from build123d import *

# Parameters (mm, degrees)
SKETCH1_W                       = 110
SKETCH1_H                       = 42
BOSS_EXTRUDE1_DEPTH             = 10
CBORE_FOR_M3_SBHCS1_D           = 3.4
CBORE_FOR_M3_SBHCS1_CBORE_D     = 8
CBORE_FOR_M3_SBHCS1_CBORE_DEPTH = 5
CUT_EXTRUDE1_DEPTH              = 10
FILLET2_R                       = 5
SKETCH6_W                       = 110
SKETCH6_H                       = 18
BOSS_EXTRUDE2_DEPTH             = 40
BOSS_EXTRUDE3_DEPTH             = 5
BOSS_EXTRUDE4_DEPTH             = 5
SKETCH10_W                      = 35
SKETCH10_H                      = 13
CUT_EXTRUDE2_DEPTH              = 15
FILLET3_R                       = 5


with BuildPart() as part:
    # Sketch1 → Boss-Extrude1 (new body)
    with BuildSketch(Plane(origin=(0, 0, 0), x_dir=(1, 0, 0), z_dir=(0, 1, 0))):
        Rectangle(SKETCH1_W, SKETCH1_H)
    extrude(amount=BOSS_EXTRUDE1_DEPTH)

    # CBORE for M3 SBHCS1 (through all)
    with Locations(Plane(origin=(0, 10, 0), x_dir=(1, 0, 0), z_dir=(0, 1, 0))):
        with Locations((-45, 8), (-32, 3), (32, 3), (45, 8)):
            CounterBoreHole(CBORE_FOR_M3_SBHCS1_D / 2, CBORE_FOR_M3_SBHCS1_CBORE_D / 2, CBORE_FOR_M3_SBHCS1_CBORE_DEPTH)

    # Sketch4 → Cut-Extrude1 (cut)
    with BuildSketch(Plane(origin=(0, 10, 0), x_dir=(1, 0, 0), z_dir=(0, 1, 0))):
        with BuildLine():
            Line((24, -21), (24, 6))
            ThreePointArc((24, 6), (22.535533906, 9.535533906), (19, 11))
            Line((19, 11), (-6, 11))
            ThreePointArc((-6, 11), (-9.535533906, 9.535533906), (-11, 6))
            Line((-11, 6), (-11, -21))
            Line((-11, -21), (24, -21))
        make_face()
    extrude(amount=-CUT_EXTRUDE1_DEPTH, mode=Mode.SUBTRACT)

    # Fillet2
    fillet2_edges = [part.edges().sort_by_distance(p)[0] for p in [
        (-11, 5, 21),
        (24, 5, 21),
    ]]
    fillet(fillet2_edges, radius=FILLET2_R)

    # Sketch6 → Boss-Extrude2 (add)
    with BuildSketch(Plane(origin=(0, 10, 0), x_dir=(1, 0, 0), z_dir=(0, 1, 0))):
        with Locations((0, -12)):
            Rectangle(SKETCH6_W, SKETCH6_H)
    extrude(amount=BOSS_EXTRUDE2_DEPTH)

    # Sketch8 → Boss-Extrude3 (add)
    with BuildSketch(Plane.ZY.offset(55)):
        Polygon((-21, 10), (3, 10), (3, 50), align=None)
    extrude(amount=-BOSS_EXTRUDE3_DEPTH)

    # Sketch9 → Boss-Extrude4 (add)
    with BuildSketch(Plane(origin=(55, 0, 0), x_dir=(0, 0, -1), z_dir=(1, 0, 0))):
        Polygon((-3, 10), (21, 10), (-3, 50), align=None)
    extrude(amount=-BOSS_EXTRUDE4_DEPTH)

    # Sketch10 → Cut-Extrude2 (cut)
    with BuildSketch(Plane.XZ.offset(-10)):
        with Locations((6.5, 9.5)):
            Rectangle(SKETCH10_W, SKETCH10_H)
    extrude(amount=-CUT_EXTRUDE2_DEPTH, mode=Mode.SUBTRACT)

    # Fillet3
    fillet3_edges = [part.edges().sort_by_distance(p)[0] for p in [
        (24, 17.5, 3),
        (6.5, 25, 3),
        (-11, 17.5, 3),
    ]]
    fillet(fillet3_edges, radius=FILLET3_R)


solid = part.part
Here's how the part is built. I have some questions about the finished solid (model axes, mm). A direction names the side the tool comes from. Coordinates: 2 decimals unless noted, no trailing zeros. Order: outer loops, then holes, each group sorted by start corner. A loop starts at its lowest first (then second) coordinate and runs counter-clockwise, first axis right, second up. Notation, with made-up numbers: M 47.5,17 L 66.5,17 A12 ccw 66.5,27 Z; hole C 23.25,86.25 d11. An arc over 180 degrees is marked long. Answer as CSV lines item,"result". Start each with the question number.
1. I want a section at B-B, the plane x = -32. Write out the boundary of the cut face in (y, z).
2. On a 3-axis mill with a long thin cutter (end or side, diameter ignored), from which of +Z, -Z, +X, -X, +Y, -Y can I reach the whole of each face in a straight line? I mean faces 4 (the flat face through (7, 5, -11)), 5 (the flat face through (-11, 7, 7)), 6 (the flat face through (6, 17, 16)), 7 (the flat face through (34, 5, -3)). Say none if no direction works.
3. I want a section at D-D, the plane z = -14.5. Write out the boundary of the cut face in (x, y), and give its area (3 significant figures).
4. I want a section at C-C, the plane y = 34. Write out the boundary of the cut face in (x, z), and give its area (3 significant figures).
5. I want a section at A-A, the plane x = 0.5. Write out the boundary of the cut face in (y, z), and give its area (3 significant figures).
6. For pin 1 (5.5 mm diameter, centred on x = 32, z = -3, fed in from +Y); pin 2 (6 mm diameter, centred on x = 36, z = 16, fed in from -Y); pin 3 (8 mm diameter, centred on x = 9, z = 3.5, fed in from -Y); pin 4 (5.5 mm diameter, centred on x = 6, z = 17.5, fed in from -Y), each with a flat end and sliding along its axis, tell me the tip position at first contact or that it passes through.
7. We'd pull the mould along Y, two halves only. Please class faces 1 (the cylindrical face through (-9, 5, -10)), 2 (the flat face through (-1, 50, 12)), 3 (the cylindrical face through (26, 18, 4)): released by +Y, released by -Y, zero draft, split by the parting line, or undercut.
8. I need wall thicknesses on line 1 (Z direction, x = 45, y = 6); line 2 (X direction, y = 7, z = 10); line 3 (X direction, y = 31.5, z = -4). Which ranges of each line are inside material? Lowest first, please. Write a range as [from, to].
Recorded:
1,outline,"M 0,-21 L 10,-21 L 10,-7 L 5,-7 L 5,-4.7 L 0,-4.7 Z; M 0,-1.3 L 5,-1.3 L 5,1 L 10,1 L 10,3 L 50,3 L 50,21 L 0,21 Z"
2,face 4,"+Z, +Y, -Y"
2,face 5,"-Y"
2,face 6,"-Z, -Y"
2,face 7,"+Y"
3,outline,"M -55,0 L 55,0 L 55,20.83 L 50,20.83 L 50,10 L -50,10 L -50,20.83 L -55,20.83 Z"
3,area,"1,210 mm2"
4,outline,"M -55,-6.6 L -50,-6.6 L -50,3 L 50,3 L 50,-6.6 L 55,-6.6 L 55,21 L -55,21 Z"
4,area,"2,080 mm2"
5,outline,"M 0,-21 L 10,-21 L 10,-11 L 0,-11 Z; M 10,16 L 25,16 L 25,8 A5 ccw 30,3 L 50,3 L 50,21 L 10,21 Z"
5,area,"620 mm2"
6,pin 1,"stops at y = 5"
6,pin 2,"stops at y = 0"
6,pin 3,"stops at y = 25.03"
6,pin 4,"stops at y = 10"
7,face 1,"zero draft"
7,face 2,"released by +Y"
7,face 3,"undercut"
8,line 1,"z = [-21, -12], [-4, 21]"
8,line 2,"x = [-55, -11], [24, 55]"
8,line 3,"x = [-55, -50], [50, 55]"
